```python
from build123d import *

# Parameters (mm, degrees)
F0_W      = 75.8
F0_H      = 35.8
F0_W_2    = 71.8000013767
F0_H_2    = 31.8
F1_DEPTH  = 5
F2_W      = 3
F2_H      = 3
F3_DEPTH  = 2
F4_R      = 5
F5_R      = 10
F6_R      = 2
F7_W      = 5
F7_H      = 2
F8_DEPTH  = 0.5
F9_W      = 5
F9_H      = 2
F10_DEPTH = 0.5
F11_SIZE  = 0.49999


# Not quite as in the source:
# - a fillet or chamfer is up to 0.001 mm smaller than in the source, because OpenCascade refuses the exact size


with BuildPart() as f1:
    # F0 (on Top) → F1 (new body)
    with BuildSketch(Plane.XY):
        with Locations((-3.8991395473, 2.3895057946)):
            Rectangle(F0_W, F0_H)
        with Locations((-3.8991395473, 2.3895057946)):
            Rectangle(F0_W_2, F0_H_2, mode=Mode.SUBTRACT)
    extrude(amount=F1_DEPTH)

    # F2 (on face) → F3 (join)
    with BuildSketch(Plane.XY.offset(5)):
        Polygon((37.0008604527, 23.2895057946), (-44.7991395473, 23.2895057946), (-44.7991395473, -18.5104942054), (34.0008604527, -18.5104942054), (34.0008604527, -15.5104942054), (37.0008604527, -15.5104942054), align=None)
        with Locations((35.5008604527, -17.0104942054)):
            Rectangle(F2_W, F2_H)
    extrude(amount=F3_DEPTH)

    # F4
    f4_edges = [f1.edges().sort_by_distance(p)[0] for p in [
        (34.00086, 20.289506, 2.5),
        (34.00086, -15.510494, 2.5),
        (-41.79914, -15.510494, 2.5),
        (-41.79914, 20.289506, 2.5),
    ]]
    fillet(f4_edges, radius=F4_R)

    # F5
    f5_edges = [f1.edges().sort_by_distance(p)[0] for p in [
        (32.000861, -13.510494, 2.5),
        (32.000861, 18.289506, 2.5),
        (-39.79914, 18.289506, 2.5),
        (-39.79914, -13.510494, 2.5),
    ]]
    fillet(f5_edges, radius=F5_R)

    # F6
    f6_edges = [f1.edges().sort_by_distance(p)[0] for p in [
        (37.00086, -18.510494, 6),
        (37.00086, 23.289506, 6),
        (-44.79914, 23.289506, 6),
        (-44.79914, -18.510494, 6),
    ]]
    fillet(f6_edges, radius=F6_R)

    # F7 (on face) → F8 (join)
    with BuildSketch(Plane(origin=(-41.7991395473, 0, 0), x_dir=(0, -1, 0), z_dir=(-1, 0, 0))):
        with Locations((-2.3895057946, 2)):
            Rectangle(F7_W, F7_H)
    extrude(amount=F8_DEPTH)

    # F9 (on face) → F10 (join)
    with BuildSketch(Plane.YZ.offset(34.0008604527)):
        with Locations((2.3895057946, 2)):
            Rectangle(F9_W, F9_H)
    extrude(amount=F10_DEPTH)

    # F11 (size 0.5 in the source; OpenCascade refuses exactly that, so slightly less here)
    f11_edges = [f1.edges().sort_by_distance(p)[0] for p in [
        (34.50086, 2.389506, 1),
        (-42.29914, 2.389506, 1),
    ]]
    chamfer(f11_edges, length=F11_SIZE)


solid = f1.part
```
For this review, take the finished solid that the model builds, in its own axes (mm). A direction names the side the tool comes from. Coordinates: 2 decimals unless noted, no trailing zeros. Loops run counter-clockwise (first coordinate to the right, second up) from the corner with the lowest first, then second, coordinate; pieces in that order, holes last. Notation, with made-up numbers: (84.5, 50) -> (132.5, 50) arc R16 ccw to (132.5, 71) -> close; hole circle Ø4 at (23, 57.5). An arc over 180 degrees is marked (long way). Return JSON: item names as keys, results as strings. Group by question number.
(1) For pin 1 Ø4 at (y, z) = (-0.5, 2.5) entering from -X; pin 2 Ø1.2 at (y, z) = (1, 2) entering from +X; pin 3 Ø5 at (x, y) = (-33.5, 2.5) entering from -Z; pin 4 Ø4 at (y, z) = (0, 3.5) entering from +X, all flat-tipped, find the tip position at first contact; note any pin that passes through.
(2) To check wall thickness, follow L1, parallel to Y at x = -28.5, z = 0.75; L2, parallel to X at y = 3.5, z = 0.75; L3, parallel to Z at x = -10, y = 8.5. State the ranges of each line that lie inside material, in increasing order.
(3) Consider section B-B, the plane y = -6.5. Give the boundary of the cut face in (x, z), plus the area to 3 significant figures.
(4) Consider section A-A, the plane x = -24.5. Give the boundary of the cut face in (y, z), plus the area to 3 significant figures.
(5) Tool access review of faces 1 (the flat face through (-4, 20.29, 2)), 2 (the flat face through (34.501, 2, 2)), 3 (the flat face through (-4, -13.51, 2)): name each direction out of +Z, -Z, +X, -X, +Y, -Y from which nothing blocks a thin tool from reaching the whole face with its end or side.
(6) Mouldability with a two-part tool opening along X and no side actions: class faces 4 (the cylindrical face through (-44.23, -17.91, 6.01)), 5 (the flat face through (37.001, 2, 6)), 6 (the cylindrical face through (29.15, 15.28, 2.54)), 7 (the cylindrical face through (28.99, -10.66, 2.54)) as pulls with the +X half, pulls with the -X half, needs draft (parallel to the pull), parting line crosses it, or undercut.
Results below:
{
 "1": {"pin 1": "stops at x = -42.3", "pin 2": "stops at x = 34.5", "pin 3": "stops at z = 5", "pin 4": "stops at x = 37"},
 "2": {"L1": "y = -15.51 to -13.51, 18.29 to 20.29", "L2": "x = -41.8 to -39.8, 32 to 34", "L3": "z = 5 to 7"},
 "3": {"outline": "(-44.8, 5) -> (-41.8, 5) -> (-41.8, 0) -> (-39.34, 0) -> (-39.34, 5) -> (31.54, 5) -> (31.54, 0) -> (34, 0) -> (34, 5) -> (37, 5) -> (37, 7) -> (-44.8, 7) -> close", "area": "188 mm2"},
 "4": {"outline": "(-18.51, 5) -> (-15.51, 5) -> (-15.51, 0) -> (-13.51, 0) -> (-13.51, 5) -> (18.29, 5) -> (18.29, 0) -> (20.29, 0) -> (20.29, 5) -> (23.29, 5) -> (23.29, 7) -> (-18.51, 7) -> close", "area": "104 mm2"},
 "5": {"face 1": "-Z, +X, -X, +Y", "face 2": "-Z, +X, +Y, -Y", "face 3": "-Z"},
 "6": {"face 4": "pulls with the -X half", "face 5": "pulls with the +X half", "face 6": "undercut", "face 7": "undercut"}
}
